Read the model definition and answer for the solid it produces. Units are mm, in the model's axes. A direction names the side the tool comes from. Coordinates: 2 decimals unless noted, no trailing zeros. Order: outer loops, then holes, each group sorted by start corner. A loop starts at its lowest first (then second) coordinate and runs counter-clockwise, first axis right, second up. Notation, with made-up numbers: (-1.5, -39) -> (20.5, -39) arc R32 cw to (20.5, -10) -> close; hole circle Ø1 at (12.25, 71). An arc over 180 degrees is marked (long way). Return JSON: item names as keys, results as strings. Group by question number.
```python
from build123d import *

# Parameters (mm, degrees)
BOSS_EXTRUDE1_DEPTH        = 3.048
BOSS_EXTRUDE2_DEPTH        = 2.032
BOSS_EXTRUDE2_DEPTH_BACK   = 47.752
BOSS_EXTRUDE2_2_DEPTH      = 2.032
BOSS_EXTRUDE2_2_DEPTH_BACK = 47.752


with BuildPart() as part:
    # Sketch1 → Boss-Extrude1 (new, symmetric)
    with BuildSketch(Plane.XY):
        with BuildLine():
            ThreePointArc((0, 27.535484012), (-9.412998127, 39.802742006), (0, 52.07))
            Line((0, 52.07), (-11.040532194, 49.111698314))
            ThreePointArc((-11.040532194, 49.111698314), (-39.066320922, 14.192289272), (-14.190605813, -23.03684931))
            Line((-14.190605813, -23.03684931), (0, -28.201807432))
            ThreePointArc((0, -28.201807432), (8.35634418, -40.135903716), (0, -52.07))
            Line((0, -52.07), (10.740686656, -48.160709762))
            ThreePointArc((10.740686656, -48.160709762), (36.144496882, -10.141220984), (7.52373904, 25.519504212))
            Line((7.52373904, 25.519504212), (0, 27.535484012))
        make_face()
        with BuildLine():
            Line((-12.7, 7.332348419), (-1.374815329, 13.870946837))
            ThreePointArc((-1.374815329, 13.870946837), (-0.410875234, 16.198104087), (1.5875, 14.664696837))
            ThreePointArc((1.5875, 14.664696837), (1.533407249, 14.253821603), (1.374815329, 13.870946837))
            Line((1.374815329, 13.870946837), (12.7, 7.332348419))
            Line((12.7, 7.332348419), (12.7, -7.332348419))
            Line((12.7, -7.332348419), (0, -14.664696837))
            Line((0, -14.664696837), (-12.7, -7.332348419))
            Line((-12.7, -7.332348419), (-12.7, 7.332348419))
        make_face(mode=Mode.SUBTRACT)
    extrude(amount=BOSS_EXTRUDE1_DEPTH, both=True)


with BuildPart() as body_2:
    # Sketch2 → Boss-Extrude2 (new, two sides: drawn at the far end of the back side and taken through both)
    with BuildSketch(Plane.XY.offset(-BOSS_EXTRUDE2_DEPTH_BACK)):
        Polygon((-70.631687067, 38.246108065), (79.453014492, 11.782125788), (82.761012277, 30.542713483), (-67.323689282, 57.00669576), align=None)
    extrude(amount=BOSS_EXTRUDE2_DEPTH + BOSS_EXTRUDE2_DEPTH_BACK)


with BuildPart() as body_3:
    # Sketch2 → Boss-Extrude2 2 (new, two sides: drawn at the far end of the back side and taken through both)
    with BuildSketch(Plane.XY.offset(-BOSS_EXTRUDE2_2_DEPTH_BACK)):
        Polygon((-79.453014492, -11.782125788), (70.631687067, -38.246108065), (67.323689282, -57.00669576), (-82.761012277, -30.542713483), align=None)
    extrude(amount=BOSS_EXTRUDE2_2_DEPTH + BOSS_EXTRUDE2_2_DEPTH_BACK)

    # Intersect1: read off the stored shape, not the designer's step
    # Intersect1: cut body 2, part
    add(body_2.part, mode=Mode.SUBTRACT)
    add(part.part, mode=Mode.SUBTRACT)


solid = body_3.part
```
1. Find section D-D on x = -9.5. Determine the outline of the cut face in (y, z).
2. For a pull along X with two mould halves and no side action, classify faces 1 (the face through (-6.67, -43.96, -23.21)), 2 (the face through (-5, -34, -47.752)), 3 (the face through (7.504, -35.562, -0.472)) as released by +X, released by -X, zero draft, split by the parting line, or undercut.
3. Straight lines are drawn through the part: L1, parallel to Z at x = 10, y = -28; L2, parallel to Y at x = -36, z = -16.5; L3, parallel to Y at x = 33, z = -34.5. For each, find the intervals that lie inside material, in ascending order.
4. Find section A-A on z = -11. Determine the outline of the cut face in (x, y).
5. Which of the six approach directions +Z, -Z, +X, -X, +Y, -Y give full straight-line access (tool end or side, diameter ignored) to faces 4 (the face through (23.01, -40.9, -0.47)), 5 (the face through (-6.512, -25.832, -0.472)), 6 (the face through (-81.13, -21.29, -23.21))?
6. Find section B-B on x = 16. Determine the outline of the cut face in (y, z), and give its area (3 significant figures).
7. Given pin 1 (1 mm diameter, centred on x = 10.5, z = -6, fed in from -Y); pin 2 (1 mm diameter, centred on x = 9, z = -12.5, fed in from +Y); pin 3 (3 mm diameter, centred on x = 16, y = -27, fed in from +Z), each flat-ended and moving along its own axis, determine where each tip first touches the part or whether it passes through.
8. Find section C-C on y = -40.5. Determine the outline of the cut face in (x, z).
Result:
{
 "1": {"outline": "(-43.46, -47.75) -> (-24.12, -47.75) -> (-24.12, -3.05) -> (-24.74, -3.05) -> (-24.74, 2.03) -> (-43.46, 2.03) -> close"},
 "2": {"face 1": "released by -X", "face 2": "zero draft", "face 3": "undercut"},
 "3": {"L1": "-47.75 to -3.05", "L2": "-38.79 to -19.44", "L3": "-50.95 to -31.61"},
 "4": {"outline": "(-82.76, -30.54) -> (67.32, -57.01) -> (70.63, -38.25) -> (-79.45, -11.78) -> close"},
 "5": {"face 4": "+Z, +Y", "face 5": "+Z, +X, +Y", "face 6": "+Z, -Z, -X, +Y"},
 "6": {"outline": "(-47.96, -47.75) -> (-28.61, -47.75) -> (-28.61, -3.05) -> (-45.79, -3.05) -> (-45.79, 2.03) -> (-47.96, 2.03) -> close", "area": "876 mm^2"},
 "7": {"pin 1": "y = -47.08", "pin 2": "y = -27.29", "pin 3": "through"},
 "8": {"outline": "(-26.29, -47.75) -> (70.23, -47.75) -> (70.23, 2.03) -> (23.46, 2.03) -> (23.46, -3.05) -> (8.35, -3.05) -> (8.35, 2.03) -> (-26.29, 2.03) -> close"}
}
